from build123d import *

# Parameters (mm, degrees)
F0_W     = 2.4
F0_H     = 4
F2_W     = 10
F2_H     = 2.052753638
F3_DEPTH = 4
F4_SIZE  = 0.5


with BuildPart() as f1:
    # F0 (on Front) → F1 (revolve)
    with BuildSketch(Plane.XZ):
        with Locations((11.2, 2)):
            Rectangle(F0_W, F0_H)
    revolve(axis=Axis((0, 0, 5.2245724946), (0, 0, 1)))

    # F2 (on face) → F3 (join, through all)
    with BuildSketch(Plane.XY.offset(4)):
        with Locations((0, 12.373623181)):
            Rectangle(F2_W, F2_H)
    extrude(amount=-F3_DEPTH)

    # F4
    f4_edges = [f1.edges().sort_by_distance(p)[0] for p in [
        (0, -12.4, 4),
        (5, 12.373623, 4),
        (0, -12.4, 0),
        (5, 12.373623, 0),
        (-5, 12.373623, 0),
        (-10, 0, 4),
        (-10, 0, 0),
    ]]
    chamfer(f4_edges, length=F4_SIZE)


solid = f1.part
The listing builds one solid part. Answer for the finished solid, in the listing's coordinates (mm). A direction names the side the tool comes from. Coordinates: 2 decimals unless noted, no trailing zeros. Write each loop counter-clockwise with the first axis right and the second up, starting at its lowest first coordinate (ties: lowest second). Pieces come first, ordered by that corner, then holes. Notation, with made-up numbers: (-6.75, 72.5) - (2.25, 72.5) arc R21 ccw to (2.25, 92.5) - close; hole circle Ø7 at (-7.75, 26). An arc over 180 degrees is marked (long way). Put each result on its own line as item: value.
1. Find the intervals of material crossed by line 1 along X through (y, z) = (0.25, 0.95); line 2 along Y through (x, z) = (0, 2.25); line 3 along X through (y, z) = (2.25, 3.3), in increasing order. Write a range as from..to.
Answer sheet:
line 1: x = -12.4..-10, 10..12.4
line 2: y = -12.4..-10, 10..13.4
line 3: x = -12.19..-9.74, 9.74..12.19
2. The part is cut by section C-C on z = 0.9. Give the vertices of the cut face in (x, y).
Answer sheet:
outline: (-5, 11.35) arc R12.4 ccw (long way) to (5, 11.35) - (5, 13.4) - (-5, 13.4) - close; hole circle Ø20 at (0, 0)
3. The part is cut by section B-B on x = 0. Give the vertices of the cut face in (y, z), plus the area to 4 significant figures.
Answer sheet:
outline: (-12.4, 0.5) - (-11.9, 0) - (-10.5, 0) - (-10, 0.5) - (-10, 3.5) - (-10.5, 4) - (-11.9, 4) - (-12.4, 3.5) - close; (10, 0.5) - (10.5, 0) - (13.4, 0) - (13.4, 4) - (10.5, 4) - (10, 3.5) - close
area: 22.45 mm^2
4. Flat-ended cylindrical pins translate along their axes: pin 1 Ø4 at (x, y) = (-9, 4) entering from -Z; pin 2 Ø1 at (y, z) = (12, 2) entering from +X; pin 3 Ø0.8 at (y, z) = (12.5, 1.5) entering from -X. Find the tip coordinate at first contact, or state that the pin passes through.
Answer sheet:
pin 1: stops at z = 0
pin 2: stops at x = 5
pin 3: stops at x = -5
5. A tool of negligible diameter and unlimited length cuts with its end or side. For faces 5 (the face through (5, 12, 2)), 6 (the face through (0, 11, 4)), from which of +Z, -Z, +X, -X, +Y, -Y can it reach the whole face along a straight path? Write none if from no direction.
Answer sheet:
face 5: +Z, -Z, +X, +Y
face 6: +Z, +X, -X, +Y, -Y
6. The part is cut by section A-A on y = 0. Give the vertices of the cut face in (x, z).
Answer sheet:
outline: (-12.4, 0.5) - (-11.9, 0) - (-10.5, 0) - (-10, 0.5) - (-10, 3.5) - (-10.5, 4) - (-11.9, 4) - (-12.4, 3.5) - close; (10, 0.5) - (10.5, 0) - (11.9, 0) - (12.4, 0.5) - (12.4, 3.5) - (11.9, 4) - (10.5, 4) - (10, 3.5) - close
7. Determine the mould class of faces 1 (the face through (-2.17, -9.76, 2.02)), 2 (the face through (0, 11, 0)), 3 (the face through (-0.47, -12.39, 2.02)), 4 (the face through (0, 13.4, 2)) for opening direction Y: pulls with the +Y half, pulls with the -Y half, needs draft (parallel to the pull), parting line crosses it, or undercut.
Answer sheet:
face 1: undercut
face 2: needs draft
face 3: parting line crosses it
face 4: pulls with the +Y half
